Work out the finished part from the listing and answer in its coordinate system (mm). A direction names the side the tool comes from. Round coordinates to 2 decimals unless told otherwise and drop trailing zeros. Loops run counter-clockwise (first coordinate to the right, second up) from the corner with the lowest first, then second, coordinate; pieces in that order, holes last. Notation, with made-up numbers: (84, -39) - (114, -39) arc R13 cw to (114, -16) - close; hole circle Ø6 at (12.25, 77). An arc over 180 degrees is marked (long way). Use CSV: the item, a comma, the result in double quotes. Start each with the question number.
from build123d import *

# Parameters (mm, degrees)
SKETCH2_W           = 184
SKETCH2_H           = 332.5
BOSS_EXTRUDE1_DEPTH = 5
SKETCH3_W           = 62.5
SKETCH3_H           = 5
SKETCH3_W_2         = 36.5
CUT_EXTRUDE2_DEPTH  = 5
CUT_EXTRUDE3_DEPTH  = 10
SKETCH5_R           = 2.1
CUT_EXTRUDE4_DEPTH  = 10
SKETCH6_R           = 2.5
CUT_EXTRUDE5_DEPTH  = 20
CUT_EXTRUDE6_DEPTH  = 10


with BuildPart() as part:
    # Sketch2 → Boss-Extrude1 (new body)
    with BuildSketch(Plane.XY):
        Rectangle(SKETCH2_W, SKETCH2_H)
    extrude(amount=BOSS_EXTRUDE1_DEPTH)

    # Sketch3 → Cut-Extrude2 (cut)
    with BuildSketch(Plane.XY.offset(5)):
        with Locations((-60.75, -98.75)):
            Rectangle(SKETCH3_W, SKETCH3_H)
        with Locations((73.75, -98.75)):
            Rectangle(SKETCH3_W_2, SKETCH3_H)
        with BuildLine():
            Line((-27.5, -141.25), (-27.5, -166.25))
            Line((-27.5, -166.25), (53.5, -166.25))
            Line((53.5, -166.25), (53.5, -141.25))
            ThreePointArc((53.5, -141.25), (13, -100.75), (-27.5, -141.25))
        make_face()
        with Locations((-60.75, 163.75)):
            Rectangle(SKETCH3_W, SKETCH3_H)
        with Locations((73.75, 163.75)):
            Rectangle(SKETCH3_W_2, SKETCH3_H)
        with Locations((-60.75, 98.75)):
            Rectangle(SKETCH3_W, SKETCH3_H)
        with Locations((73.75, 98.75)):
            Rectangle(SKETCH3_W_2, SKETCH3_H)
    extrude(amount=-CUT_EXTRUDE2_DEPTH, mode=Mode.SUBTRACT)

    # Sketch4 → Cut-Extrude3 (cut)
    with BuildSketch(Plane.XY.offset(5)):
        Polygon((-55.75, 161.25), (-55.75, 151.25), (-58.65, 151.25), (-58.65, 146.25), (-62.85, 146.25), (-62.85, 151.25), (-65.75, 151.25), (-65.75, 161.25), align=None)
        Polygon((78.75, 161.25), (78.75, 151.25), (75.85, 151.25), (75.85, 146.25), (71.65, 146.25), (71.65, 151.25), (68.75, 151.25), (68.75, 161.25), align=None)
        Polygon((68.75, -166.25), (68.75, -156.25), (71.65, -156.25), (71.65, -151.25), (75.85, -151.25), (75.85, -156.25), (78.75, -156.25), (78.75, -166.25), align=None)
        Polygon((-65.75, -166.25), (-65.75, -156.25), (-62.85, -156.25), (-62.85, -151.25), (-58.65, -151.25), (-58.65, -156.25), (-55.75, -156.25), (-55.75, -166.25), align=None)
    extrude(amount=-CUT_EXTRUDE3_DEPTH, mode=Mode.SUBTRACT)

    # Sketch5 → Cut-Extrude4 (cut)
    with BuildSketch(Plane.XY.offset(5)):
        with Locations((13, 98.75)):
            Circle(SKETCH5_R)
    extrude(amount=-CUT_EXTRUDE4_DEPTH, mode=Mode.SUBTRACT)

    # Sketch6 → Cut-Extrude5 (cut)
    with BuildSketch(Plane(origin=(0, 0, 0), x_dir=(-1, 0, 0), z_dir=(0, 0, -1))):
        with Locations((35.2, -111.17)):
            Circle(SKETCH6_R)
        with Locations((35.2, -121.33)):
            Circle(SKETCH6_R)
        with Locations((84.2, -121.33)):
            Circle(SKETCH6_R)
        with Locations((84.2, -111.17)):
            Circle(SKETCH6_R)
        Polygon((40.7, -106.25), (40.399667757, -106.296165348), (40.234631653, -106.364882888), (40.087708911, -106.459367581), (39.992893219, -106.542893219), (39.859754352, -106.707794088), (39.773544355, -106.873596044), (39.723897446, -107.032689615), (39.7, -107.25), (39.7, -125.25), (39.821493713, -125.727730786), (39.992893219, -125.957106781), (40.299461949, -126.166280126), (40.7, -126.25), (78.2, -126.25), (78.7, -126.25), (79.000332243, -126.203834652), (79.284083673, -126.061693454), (79.431556814, -125.931780484), (79.678284878, -125.4572648), (79.7, -125.25), (79.7, -107.25), (79.694079498, -107.141344807), (79.68082013, -107.055084963), (79.654773565, -106.952666114), (79.626455645, -106.873596044), (79.58827866, -106.790695066), (79.540245648, -106.707794088), (79.480899769, -106.625343654), (79.431556814, -106.568219516), (79.407106781, -106.542893219), (79.357820244, -106.496825036), (79.297626381, -106.448225275), (79.228612143, -106.401136523), (79.142207958, -106.35308745), (79.088762914, -106.32866217), (79.000332243, -106.296165348), (78.955551566, -106.283204573), (78.853081535, -106.261786438), (78.755064535, -106.251517202), (78.7, -106.25), align=None)
    extrude(amount=-CUT_EXTRUDE5_DEPTH, mode=Mode.SUBTRACT)

    # Sketch7 → Cut-Extrude6 (cut)
    with BuildSketch(Plane(origin=(0, 0, 0), x_dir=(-1, 0, 0), z_dir=(0, 0, -1))):
        with BuildLine():
            Line((92.154047247, -4.010729367), (92, -22.885338591))
            ThreePointArc((92, -22.885338591), (64.618518363, -14.841480585), (36.080546525, -14.658856257))
            ThreePointArc((36.080546525, -14.658856257), (37.397553955, -5.515336457), (39.976105832, 3.355375641))
            ThreePointArc((39.976105832, 3.355375641), (66.474403295, 2.571796797), (92.154047247, -4.010729367))
        make_face()
    extrude(amount=-CUT_EXTRUDE6_DEPTH, mode=Mode.SUBTRACT)


solid = part.part
Item 1: A cutting plane is placed at B-B (z = 2.1). State how many separate pieces and enclosed holes the cut face has, plus the area to 3 significant figures.
Item 2: A cutting plane is placed at A-A (x = 62). Determine the outline of the cut face in (y, z), plus the area to 3 significant figures.
Item 3: The mould has two halves that part along Y. Classify faces 1 (the cylindrical face through (-65, -14.9, 2.5)), 2 (the cylindrical face through (13.89, -100.76, 2.54)), 3 (the flat face through (-1, 2, 5)): pulls with the +Y half, pulls with the -Y half, needs draft (parallel to the pull), parting line crosses it, or undercut.
Item 4: A cutting plane is placed at C-C (x = 25). Determine the outline of the cut face in (y, z).
Item 5: Each of these flat-tipped pins is pushed along its axis until it touches: pin 1 Ø1.3 at (x, z) = (-61.5, 2) entering from -Y; pin 2 Ø1.4 at (x, z) = (-63.5, 3.5) entering from -Y; pin 3 Ø2.5 at (y, z) = (164.5, 3.5) entering from -X. Where does it stop, or does it pass through?
Item 6: A cutting plane is placed at D-D (x = -11.5). Determine the outline of the cut face in (y, z).
Item 7: Which of the six approach directions +Z, -Z, +X, -X, +Y, -Y give full straight-line access (tool end or side, diameter ignored) to faces 4 (the flat face through (-1, 2, 0)), 5 (the cylindrical face through (-66.026, 2.634, 2.465))?
Item 8: Find the intervals of material crossed by probe 1 along Y at (x, z) = (-35.2, 2.8); probe 2 along Y at (x, z) = (-52, 3.9); probe 3 along Y at (x, z) = (68.5, 4.85), in increasing order. Write a range as [from, to].
Result sheet:
1,separate pieces,"1"
1,enclosed holes,"6"
1,area,"52,700 mm^2"
2,outline,"(-166.25, 0) - (-101.25, 0) - (-101.25, 5) - (-166.25, 5) - close; (-96.25, 0) - (96.25, 0) - (96.25, 5) - (-96.25, 5) - close; (101.25, 0) - (161.25, 0) - (161.25, 5) - (101.25, 5) - close"
2,area,"1,590 mm^2"
3,face 1,"undercut"
3,face 2,"pulls with the -Y half"
3,face 3,"needs draft"
4,outline,"(-102.57, 0) - (166.25, 0) - (166.25, 5) - (-102.57, 5) - close"
5,pin 1,"y = -151.25"
5,pin 2,"y = -156.25"
5,pin 3,"x = -29.5"
6,outline,"(-109, 0) - (166.25, 0) - (166.25, 5) - (-109, 5) - close"
7,face 4,"-Z, +X, -X, +Y, -Y"
7,face 5,"+Z, -Z"
8,probe 1,"[-166.25, -123.83], [-118.83, -113.67], [-108.67, -101.25], [-96.25, 96.25], [101.25, 161.25]"
8,probe 2,"[-166.25, -126.25], [-106.25, -101.25], [-96.25, -13.78], [3.73, 96.25], [101.25, 161.25]"
8,probe 3,"[-166.25, -101.25], [-96.25, 96.25], [101.25, 161.25]"
